Source: three-view drawing plus pictorial views. Frame: mm from the lowest corner of the part. A direction names the side the tool comes from. Give positions to 0.01 mm unless a question says otherwise; leave off trailing zeros. Write each loop counter-clockwise with the first axis right and the second up, starting at its lowest first coordinate (ties: lowest second). Pieces come first, ordered by that corner, then holes. Notation, with made-up numbers: (68, 20) -> (123, 20) arc R23 cw to (123, 51) -> close; hole circle Ø3 at (47, -16). An arc over 180 degrees is marked (long way). Use a Markdown table: item, result. Add a question column.
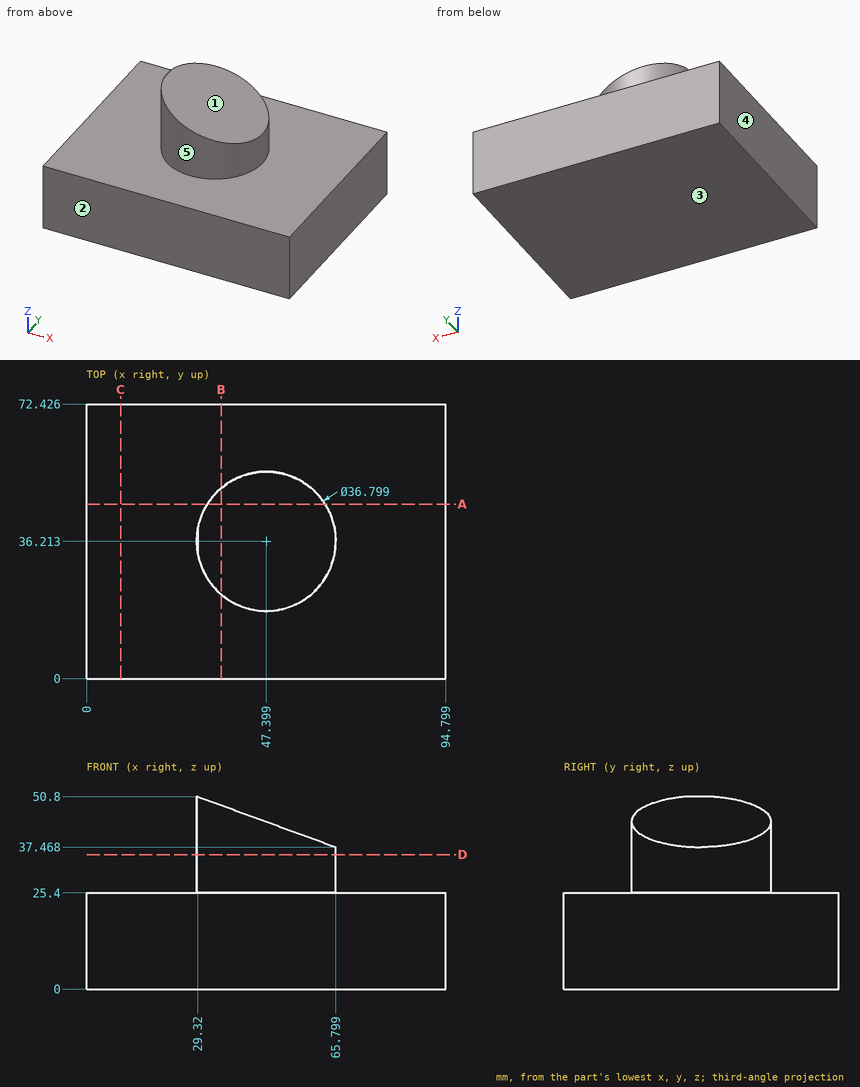
(1) Mould query, pull axis Z, two halves, no side actions, for the marked faces 1, 2 and 3. Classes: +Z half, -Z half, draft (parallel to the pull), parting line (faces both ways), or undercut.
(2) Cut plane D-D on z = 35.5. Return the cut outline in (x, y).
(3) Cut plane A-A on y = 46. Return the cut outline in (x, z).
(4) Cut plane C-C on x = 9. Return the cut outline in (y, z).
(5) Cut plane B-B on x = 35.5. Return the cut outline in (y, z).
(6) Access query for the marked faces 4 and 5. Directions: +Z, -Z, +X, -X, +Y, -Y. A direction counts if a zero-diameter tool reaches every point of the face in a straight line with its end or side. Return the directions, or none.
(7) Material intervals for L1, parallel to Z at x = 7, y = 64; L2, parallel to Z at x = 45.5, y = 26; L3, parallel to X at y = 28.5, z = 31 (1 decimal), sorted ascending.
(8) First-contact query: pin 1 Ø2 at (x, z) = (55, 14) entering from -Y; pin 2 Ø5 at (x, y) = (62, 62) entering from +Z; pin 3 Ø10 at (x, z) = (40.5, 31.5) entering from +Y (1 decimal). Flat tips, straight axial feed; report the tip coordinate or a pass-through.
Output:
| question | item | result |
|---|---|---|
| 1 | face 1 | +Z half |
| 1 | face 2 | draft |
| 1 | face 3 | -Z half |
| 2 | outline | circle Ø36.8 at (47.4, 36.21) |
| 3 | outline | (0, 0) -> (94.8, 0) -> (94.8, 25.4) -> (62.98, 25.4) -> (62.98, 38.5) -> (31.82, 49.89) -> (31.82, 25.4) -> (0, 25.4) -> close |
| 4 | outline | (0, 0) -> (72.43, 0) -> (72.43, 25.4) -> (0, 25.4) -> close |
| 5 | outline | (0, 0) -> (72.43, 0) -> (72.43, 25.4) -> (50.25, 25.4) -> (50.25, 48.54) -> (22.18, 48.54) -> (22.18, 25.4) -> (0, 25.4) -> close |
| 6 | face 4 | +Z, -Z, -X, +Y, -Y |
| 6 | face 5 | +Z |
| 7 | L1 | 0 to 25.4 |
| 7 | L2 | 0 to 44.89 |
| 7 | L3 | 30.7 to 64.1 |
| 8 | pin 1 | y = 0 |
| 8 | pin 2 | z = 25.4 |
| 8 | pin 3 | y = 54.5 |
